CAD build for the part. Positions are in the model's coordinates, mm. Face numbers are marked on the shaded views. A direction names the side the tool comes from. Round coordinates to 2 decimals unless told otherwise and drop trailing zeros.
from build123d import *

# Parameters (mm, degrees)
F0_W     = 360
F0_H     = 470
F1_DEPTH = 235
F1_TAPER = 5
F2_T     = -10


with BuildPart() as f1:
    # F0 (on Top) → F1 (new body)
    with BuildSketch(Plane.XY):
        Rectangle(F0_W, F0_H)
    extrude(amount=-F1_DEPTH, taper=F1_TAPER)

    # F2
    f2_openings = [f1.faces().sort_by_distance(p)[0] for p in [
        (0, 0, 0),
    ]]
    offset(amount=F2_T, openings=f2_openings, kind=Kind.INTERSECTION)


solid = f1.part
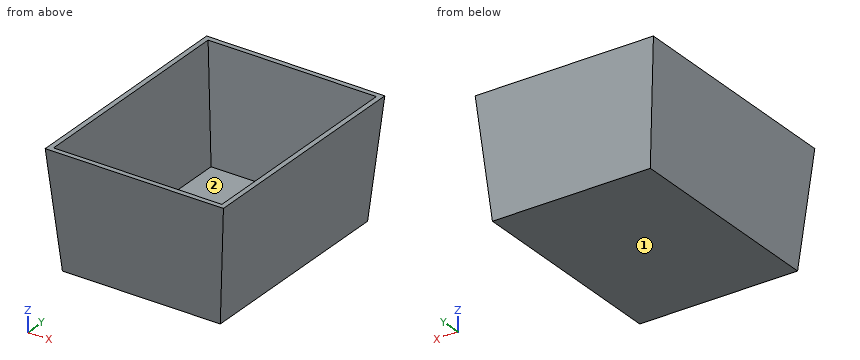
Item 1: 3-axis set-ups, long thin cutter, end or side, ignore diameter. For the marked faces 1 and 2: which of +Z, -Z, +X, -X, +Y, -Y reach the whole face in a straight line?
Verdict:
face 1: -Z, +X, -X, +Y, -Y
face 2: +Z
Item 2: Flat gauge pins, fed straight in: P1, Ø3, axis at y = -140.5, z = -37, coming from the +X side; P2, Ø1, axis at x = -117.5, z = -88, coming from the +Y side; P3, Ø12, axis at x = -121, z = -145, coming from the +Y side. Where does each tip first touch, or does it go through?
Verdict:
P1: stops at x = 176.89
P2: stops at y = 227.34
P3: stops at y = 222.84
Item 3: Wall check: L1, parallel to Z at x = 99.5, y = -37.5; L2, parallel to Y at x = 65.5, z = -63; L3, parallel to Y at x = -30, z = -93.5. Give the ranges that are in metal, low to high.
Verdict:
L1: z = -235 to -225
L2: y = -229.49 to -219.45, 219.45 to 229.49
L3: y = -226.82 to -216.78, 216.78 to 226.82
